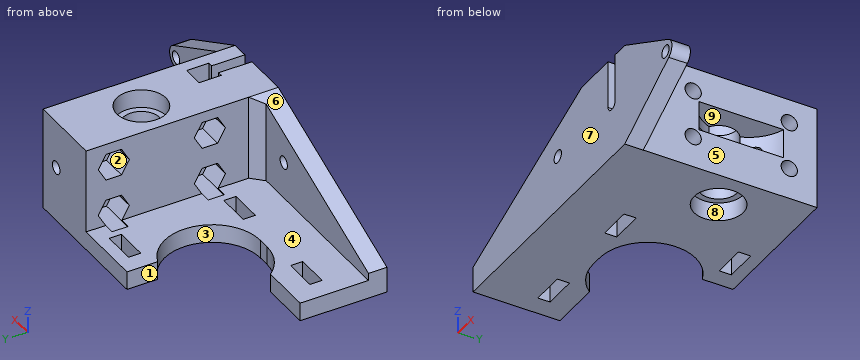
from build123d import *

# Parameters (mm, degrees)
SKETCH1_R               = 5
SKETCH1_W               = 9
SKETCH1_H               = 3.3
BOSS_EXTRUDE1_DEPTH     = 28
SKETCH2_W               = 50.5
SKETCH2_H               = 47
CUT_EXTRUDE1_DEPTH      = 23
SKETCH3_R               = 6.65
CUT_EXTRUDE2_DEPTH      = 5
CUT_EXTRUDE3_START      = -5
SKETCH4_R               = 6.65
CUT_EXTRUDE3_DEPTH      = 5
SKETCH5_R               = 12
CUT_EXTRUDE4_DEPTH      = 8
CUT_EXTRUDE5_START      = -9
CUT_EXTRUDE5_DEPTH      = 9
CUT_EXTRUDE6_DEPTH      = 6
SKETCH8_R               = 1.15
CUT_EXTRUDE7_DEPTH      = 85.190260719
CHAMFER1_SIZE           = 21
CHAMFER1_SIZE2          = 50.5
SKETCH9_R               = 2.2
CUT_EXTRUDE8_DEPTH      = 83.137080542
CUT_EXTRUDE9_DEPTH      = 3
CUT_EXTRUDE9_DEPTH_BACK = 7
SKETCH12_R              = 1.75
CUT_EXTRUDE10_DEPTH     = 10
CHAMFER2_SIZE           = 3
BOSS_EXTRUDE3_DEPTH     = 5
SKETCH15_R              = 1.7
CUT_EXTRUDE11_DEPTH     = 85.190260719


with BuildPart() as part:
    # Sketch1 → Boss-Extrude1 (new body)
    with BuildSketch(Plane.XY):
        with BuildLine():
            Line((-60, -31.5), (10.5, -31.5))
            Line((10.5, -31.5), (10.5, 20.5))
            Line((10.5, 20.5), (-28.5, 20.5))
            Line((-28.5, 20.5), (-28.5, 12.180409823))
            ThreePointArc((-28.5, 12.180409823), (-20.217668105, -2.285689125), (-33, -12.985083113))
            Line((-33, -12.985083113), (-36, -12.985083113))
            ThreePointArc((-36, -12.985083113), (-41.689100041, -11.672468641), (-46.228019527, -8))
            Line((-46.228019527, -8), (-60, -8))
            Line((-60, -8), (-60, -31.5))
        make_face()
        Circle(SKETCH1_R, mode=Mode.SUBTRACT)
        with Locations((-19, 15.5)):
            Rectangle(SKETCH1_W, SKETCH1_H, mode=Mode.SUBTRACT)
        with Locations((-19, -15.5)):
            Rectangle(SKETCH1_W, SKETCH1_H, mode=Mode.SUBTRACT)
        with Locations((-50, -15.5)):
            Rectangle(SKETCH1_W, SKETCH1_H, mode=Mode.SUBTRACT)
    extrude(amount=BOSS_EXTRUDE1_DEPTH)

    # Sketch2 → Cut-Extrude1 (cut)
    with BuildSketch(Plane.XY.offset(28)):
        with Locations((-34.75, -3)):
            Rectangle(SKETCH2_W, SKETCH2_H)
    extrude(amount=-CUT_EXTRUDE1_DEPTH, mode=Mode.SUBTRACT)

    # Sketch3 → Cut-Extrude2 (cut)
    with BuildSketch(Plane.XY.offset(28)):
        Circle(SKETCH3_R)
    extrude(amount=-CUT_EXTRUDE2_DEPTH, mode=Mode.SUBTRACT)

    # Sketch4 → Cut-Extrude3 (cut)
    with BuildSketch(Plane(origin=(0, 0, 0), x_dir=(-1, 0, 0), z_dir=(0, 0, -1)).offset(CUT_EXTRUDE3_START)):
        with Locations(Location((0, 0, 0), (0, 0, 180))):
            Circle(SKETCH4_R)
    extrude(amount=CUT_EXTRUDE3_DEPTH, mode=Mode.SUBTRACT)

    # Sketch5 → Cut-Extrude4 (cut)
    with BuildSketch(Plane.XY.offset(11)):
        with Locations((14, 0)):
            Circle(SKETCH5_R)
    extrude(amount=CUT_EXTRUDE4_DEPTH, mode=Mode.SUBTRACT)

    # Sketch6 → Cut-Extrude5 (cut)
    with BuildSketch(Plane.XZ.offset(31.5).offset(CUT_EXTRUDE5_START)):
        with BuildLine():
            Line((2.725, 15), (2.725, 28))
            Line((2.725, 28), (6.025, 28))
            Line((6.025, 28), (6.025, 15))
            ThreePointArc((6.025, 15), (4.375, 13.35), (2.725, 15))
        make_face()
    extrude(amount=CUT_EXTRUDE5_DEPTH, mode=Mode.SUBTRACT)

    # Sketch7 → Cut-Extrude6 (cut)
    with BuildSketch(Plane.XZ.offset(22.5)):
        Polygon((1.475, 28), (7.275, 28), (7.275, 13.325684219), (4.375, 11.651368439), (1.475, 13.325684219), align=None)
    extrude(amount=-CUT_EXTRUDE6_DEPTH, mode=Mode.SUBTRACT)

    # Sketch8 → Cut-Extrude7 (cut, through all)
    with BuildSketch(Plane.XZ.offset(31.5)):
        with Locations(Location((4.375, 15, 0), (0, 0, 270))):
            Circle(SKETCH8_R)
    extrude(amount=-CUT_EXTRUDE7_DEPTH, mode=Mode.SUBTRACT)

    # Chamfer1
    chamfer1_edges = [part.edges().sort_by_distance(p)[0] for p in [
        (-60, -29, 28),
    ]]
    chamfer1_side = [part.faces().sort_by_distance(p)[0] for p in [
        (-60, -19.75, 0.365547535),
    ]]
    chamfer(chamfer1_edges, length=CHAMFER1_SIZE, length2=CHAMFER1_SIZE2, reference=chamfer1_side[0])

    # Sketch9 → Cut-Extrude8 (cut, through all)
    with BuildSketch(Plane(origin=(10.5, 0, 0), x_dir=(0, 0, -1), z_dir=(1, 0, 0))):
        with Locations((-8.5, 13)):
            Circle(SKETCH9_R)
        with Locations(Location((-21.5, 13, 0), (0, 0, 90))):
            Circle(SKETCH9_R)
        with Locations(Location((-8.5, -13, 0), (0, 0, 90))):
            Circle(SKETCH9_R)
        with Locations((-21.5, -13)):
            Circle(SKETCH9_R)
    extrude(amount=-CUT_EXTRUDE8_DEPTH, mode=Mode.SUBTRACT)

    # Sketch10 → Cut-Extrude9 (cut, two sides: drawn at the far end of the back side and taken through both)
    with BuildSketch(Plane.ZY.offset(9.5).offset(-CUT_EXTRUDE9_DEPTH_BACK)):
        Polygon((4.85, 15.107328483), (4.85, 10.892671517), (8.5, 8.785343035), (12.15, 10.892671517), (12.15, 15.107328483), (8.5, 17.214656965), align=None)
        Polygon((25.15, 10.892671517), (25.15, 15.107328483), (21.5, 17.214656965), (17.85, 15.107328483), (17.85, 10.892671517), (21.5, 8.785343035), align=None)
        Polygon((25.15, -10.892671517), (21.5, -8.785343035), (17.85, -10.892671517), (17.85, -15.107328483), (21.5, -17.214656965), (25.15, -15.107328483), align=None)
        Polygon((12.15, -10.892671517), (8.5, -8.785343035), (4.85, -10.892671517), (4.85, -15.107328483), (8.5, -17.214656965), (12.15, -15.107328483), align=None)
    extrude(amount=CUT_EXTRUDE9_DEPTH + CUT_EXTRUDE9_DEPTH_BACK, mode=Mode.SUBTRACT)

    # Sketch12 → Cut-Extrude10 (cut)
    with BuildSketch(Plane(origin=(0, 20.5, 0), x_dir=(1, 0, 0), z_dir=(0, 1, 0))):
        with Locations(Location((4.375, -15, 0), (0, 0, 270))):
            Circle(SKETCH12_R)
    extrude(amount=-CUT_EXTRUDE10_DEPTH, mode=Mode.SUBTRACT)

    # Chamfer2
    chamfer2_edges = [part.edges().sort_by_distance(p)[0] for p in [
        (-9.5, -26.5, 16.5),
    ]]
    chamfer(chamfer2_edges, length=CHAMFER2_SIZE)

    # Sketch14 → Boss-Extrude3 (add)
    with BuildSketch(Plane.XZ.offset(31.5)):
        with BuildLine():
            Line((10.5, 0), (30.934731544, 12.437337808))
            ThreePointArc((30.934731544, 12.437337808), (32.372897026, 15.112309482), (30.73861997, 17.672178994))
            Line((30.73861997, 17.672178994), (10.5, 28))
            Line((10.5, 28), (10.5, 0))
        make_face()
    extrude(amount=-BOSS_EXTRUDE3_DEPTH)

    # Sketch15 → Cut-Extrude11 (cut, through all)
    with BuildSketch(Plane.XZ.offset(31.5)):
        with Locations(Location((-20.625, 15, 0), (0, 0, 270))):
            Circle(SKETCH15_R)
        with Locations(Location((29.375, 15, 0), (0, 0, 270))):
            Circle(SKETCH15_R)
    extrude(amount=-CUT_EXTRUDE11_DEPTH, mode=Mode.SUBTRACT)


solid = part.part
Source: CAD feature listing. Evaluate the final solid. Frame: model axes, mm. Face numbers are marked on the shaded views. A direction names the side the tool comes from. Give positions to 0.01 mm unless a question says otherwise; leave off trailing zeros. Order: outer loops, then holes, each group sorted by start corner. A loop starts at its lowest first (then second) coordinate and runs counter-clockwise, first axis right, second up. Notation, with made-up numbers: (-31.5, 87.25) -> (-13.5, 87.25) arc R16 cw to (-13.5, 105.25) -> close; hole circle Ø8 at (66, 36). An arc over 180 degrees is marked (long way). Write item = value, one per line.
Q1. Set-up query: the marked faces 1, 2, 3, 4 and 5. Return all of +Z, -Z, +X, -X, +Y, -Y with unobstructed straight access to the full face (end or side cutting, diameter ignored); none if empty.
Data:
face_1 = +Z, -Z, -X, +Y
face_2 = -X
face_3 = +Z, -Z
face_4 = +Z, -X, +Y
face_5 = +Z, -Z, +X, +Y
Q2. Cut plane D-D, the plane z = 3. Output: boundary loops of the cut face in (x, y).
Data:
outline = (-60, -31.5) -> (15.43, -31.5) -> (15.43, -26.5) -> (10.5, -26.5) -> (10.5, 20.5) -> (-28.5, 20.5) -> (-28.5, 12.18) arc R12.99 cw to (-33, -12.99) -> (-36, -12.99) arc R12.99 cw to (-46.23, -8) -> (-60, -8) -> close; hole (-54.5, -17.15) -> (-45.5, -17.15) -> (-45.5, -13.85) -> (-54.5, -13.85) -> close; hole (-23.5, -17.15) -> (-14.5, -17.15) -> (-14.5, -13.85) -> (-23.5, -13.85) -> close; hole (-23.5, 13.85) -> (-14.5, 13.85) -> (-14.5, 17.15) -> (-23.5, 17.15) -> close; hole circle Ø13.3 at (0, 0)
Q3. Material intervals for line 1 (Z direction, x = -4.5, y = 13); line 2 (X direction, y = -21.5, z = 26) (3 decimals); line 3 (Y direction, x = -52, z = 4), sorted ascending. Write a range as from..to.
Data:
line_1 = 0..4.85, 12.15..17.85, 25.15..28
line_2 = -9.5..1.475, 7.275..10.5
line_3 = -31.5..-17.15, -13.85..-8
Q4. Pin query (flat end, axial travel): pin 1 (1 mm diameter, centred on y = -9.5, z = 9.5, fed in from +X); pin 2 (1.5 mm diameter, centred on y = -12.5, z = 7, fed in from -X); pin 3 (1.5 mm diameter, centred on y = 16.5, z = 3.5, fed in from -X). Return the tip coordinate at first contact, or that it passes through.
Data:
pin_1 = 10.5
pin_2 = -2.5
pin_3 = -28.5
Q5. Cut plane C-C, the plane x = -16.5. Output: boundary loops of the cut face in (y, z).
Data:
outline = (-31.5, 0) -> (-17.15, 0) -> (-17.15, 5) -> (-26.5, 5) -> (-26.5, 25.09) -> (-31.5, 25.09) -> close; (-13.85, 0) -> (13.85, 0) -> (13.85, 5) -> (-13.85, 5) -> close; (17.15, 0) -> (20.5, 0) -> (20.5, 5) -> (17.15, 5) -> close
Q6. Cut plane A-A, the plane z = 20.25. State how many separate pieces and enclosed holes the cut face has, and give its area (3 significant figures).
Data:
separate_pieces = 3
enclosed_holes = 1
area = 879 mm^2
Q7. Pull-direction query (Y, two-part tool) for the marked faces 6, 7, 8 and 9; classes: released by +Y, released by -Y, zero draft, split by the parting line, or undercut.
Data:
face_6 = zero draft
face_7 = released by -Y
face_8 = undercut
face_9 = undercut
Q8. Cut plane B-B, the plane y = 0. Output: boundary loops of the cut face in (x, z).
Data:
outline = (-20.01, 0) -> (-6.65, 0) -> (-6.65, 5) -> (-5, 5) -> (-5, 23) -> (-6.65, 23) -> (-6.65, 28) -> (-9.5, 28) -> (-9.5, 5) -> (-20.01, 5) -> close; (5, 5) -> (6.65, 5) -> (6.65, 0) -> (10.5, 0) -> (10.5, 11) -> (5, 11) -> close; (5, 19) -> (10.5, 19) -> (10.5, 28) -> (6.65, 28) -> (6.65, 23) -> (5, 23) -> close
